Autodesk Inventor part; units mm, degrees
ref_plane "YZ Plane" through (0, 0, 0) normal (1, 0, 0) x (0, 1, 0)
ref_plane "XZ Plane" through (0, 0, 0) normal (0, 1, 0) x (-1, 0, 0)
ref_plane "XY Plane" through (0, 0, 0) normal (0, 0, 1) x (1, 0, 0)
sketch "Эскиз1" plane through (0, 0, 0) normal (0, 0, 1) x (1, 0, 0)
  line L0 (20, -18.5) -> (20, -13.95) construction
  line L1 (-240, -18.5) -> (20, -18.5) construction
  line L2 (20, -18.5) -> (-40, -18.5)
  line L3 (-40, -18.5) -> (-40, 5.5)
  line L4 (-40, 5.5) -> (20, 5.5)
  line L5 (20, 5.5) -> (20, -18.5)
  point P0 (0, 0)
  dimension "d0" = 60
  dimension "d1" = 24
extrude "Выдавливание1" add sketch "Эскиз1" along normal blind 4
fillet "Сопряжение1" radius 4 4 edges at (-40, 5.5, 2) (-40, -18.5, 2) (20, -18.5, 2) (20, 5.5, 2)
sketch "Эскиз2" plane through (0, 0, 4) normal (0, 0, 1) x (1, 0, 0)
  circle A0 centre (-21, 219) radius 7.5 construction
  line L0 (-21, 219) -> (-21, -6.68) construction
  arc A1 (-40, -14.5) -> (-36, -18.5) centre (-36, -14.5) ccw construction
  arc A2 (20, 1.5) -> (16, 5.5) centre (16, 1.5) ccw construction
  line L1 (-10, -6.5) -> (-40, -6.5) construction
  line L2 (-240, -6.68) -> (20, -6.68) construction
  line L3 (-240, -13.32) -> (20, -13.32) construction
  line L4 (-21, -6.68) -> (-21, -13.32) construction
  line L5 (-21, -13.32) -> (-21, -31) construction
  circle A3 centre (-21, -10) radius 2.5
  circle A4 centre (-5.5, -10) radius 2
  circle A5 centre (10, -10) radius 2
  line L6 (20, -14.5) -> (20, 1.5)
  point P0 (0, 0)
  dimension "d5" = 250
  dimension "d6" = 5
  dimension "d7" = 4
  dimension "d8" = 4
  dimension "d9" = 10
  dimension "d10" = 15.5
extrude "Выдавливание2" cut sketch "Эскиз2" against normal blind 4
properties part number "креп. пасс. ролика"
Can you work these out from the model? Positions are in its coordinate system, mm. Coordinates: 2 decimals unless noted, no trailing zeros. Loops run counter-clockwise (first coordinate to the right, second up) from the corner with the lowest first, then second, coordinate; pieces in that order, holes last. Notation, with made-up numbers: (-23.75, 74.25) - (28.25, 74.25) arc R30 cw to (28.25, 108.25) - close; hole circle Ø8 at (-9.5, 38). An arc over 180 degrees is marked (long way). Use a Markdown table: item, result.
Item 1: I want a section at C-C on z = 1. Please give me the cut outline in (x, y).
Numbers:
| item | result |
|---|---|
| outline | (-40, -14.5) arc R4 ccw to (-36, -18.5) - (16, -18.5) arc R4 ccw to (20, -14.5) - (20, 1.5) arc R4 ccw to (16, 5.5) - (-36, 5.5) arc R4 ccw to (-40, 1.5) - close; hole circle Ø5 at (-21, -10); hole circle Ø4 at (-5.5, -10); hole circle Ø4 at (10, -10) |
Item 2: If I drill on probe 1 along Y at (x, z) = (-19.5, 1.4); probe 2 along Y at (x, z) = (-21, 1.8); probe 3 along X at (y, z) = (-9.75, 1.1), over which ranges is the centre line in solid material (lowest first)? Write a range as from..to.
Numbers:
| item | result |
|---|---|
| probe 1 | y = -18.5..-12, -8..5.5 |
| probe 2 | y = -18.5..-12.5, -7.5..5.5 |
| probe 3 | x = -40..-23.49, -18.51..-7.48, -3.52..8.02, 11.98..20 |
Item 3: I want a section at A-A on x = -21. Please give me the cut outline in (y, z).
Numbers:
| item | result |
|---|---|
| outline | (-18.5, 0) - (-12.5, 0) - (-12.5, 4) - (-18.5, 4) - close; (-7.5, 0) - (5.5, 0) - (5.5, 4) - (-7.5, 4) - close |
Item 4: We'd pull the mould along X, two halves only. Please class faces 1 (the face through (-38.859, -17.297, 2.028)), 2 (the face through (-10, -6, 4)), 3 (the face through (-23, -11.5, 2)): released by +X, released by -X, zero draft, split by the parting line, or undercut.
Numbers:
| item | result |
|---|---|
| face 1 | released by -X |
| face 2 | zero draft |
| face 3 | undercut |
Item 5: I want a section at D-D on x = -5.5. Please give me the cut outline in (y, z).
Numbers:
| item | result |
|---|---|
| outline | (-18.5, 0) - (-12, 0) - (-12, 4) - (-18.5, 4) - close; (-8, 0) - (5.5, 0) - (5.5, 4) - (-8, 4) - close |
Item 6: I want a section at B-B on y = -10. Please give me the cut outline in (x, z).
Numbers:
| item | result |
|---|---|
| outline | (-40, 0) - (-23.5, 0) - (-23.5, 4) - (-40, 4) - close; (-18.5, 0) - (-7.5, 0) - (-7.5, 4) - (-18.5, 4) - close; (-3.5, 0) - (8, 0) - (8, 4) - (-3.5, 4) - close; (12, 0) - (20, 0) - (20, 4) - (12, 4) - close |
